Verification items for the finished model (mm, model axes). Face numbers are marked on the shaded views. A direction names the side the tool comes from. Round coordinates to 2 decimals unless told otherwise and drop trailing zeros. Write each loop counter-clockwise with the first axis right and the second up, starting at its lowest first coordinate (ties: lowest second). Pieces come first, ordered by that corner, then holes. Notation, with made-up numbers: M -17.75,3 L -6.75,3 A28 cw -6.75,41 Z; hole C 77.5,12 d9. An arc over 180 degrees is marked long. One line per item, written item: value. Start each with the question number.
from build123d import *

# Parameters (mm, degrees)
BASE_FLANGE1_DEPTH             = 7.62
EDGE_FLANGE1_STRIP_W           = 12.7
EDGE_FLANGE1_STRIP_H           = 1.5875
EDGE_FLANGE1_STRIP_CUT_DEPTH   = 13.689174868
EDGE_FLANGE1_STRIP_2_W         = 12.7
EDGE_FLANGE1_STRIP_2_H         = 1.5875
EDGE_FLANGE1_STRIP_CUT_2_DEPTH = 13.689174868
EDGE_FLANGE1_DEPTH             = 13.689174868
EDGE_FLANGE1_BEND_DEPTH        = 13.689174868
SKETCH12_W                     = 0.396875
SKETCH12_H                     = 4.784490506
SKETCH12_H_2                   = 4.782978668
CUT_EXTRUDE3_DEPTH             = 25.4
SKETCH13_W                     = 0.396875
SKETCH13_H                     = 4.7625
CUT_EXTRUDE4_DEPTH             = 25.4
FILLET2_R                      = 0.79375
BOSS_EXTRUDE1_DEPTH            = 1.5875
FILLET3_R                      = 3.175
FILLET4_R                      = 4.7625
FILLET5_R                      = 0.79375


# Read off the part's stored shape, not the designer's step: Base-Flange1
# Sheet-metal steps are written as plain solids
with BuildPart() as part:
    # Base-Flange1 outline → Base-Flange1 (new body)
    with BuildSketch(Plane(origin=(0, 0, 0), x_dir=(1, 0, 0), z_dir=(0, 1, 0))):
        with BuildLine():
            ThreePointArc((24.665208878, -10.952288676), (26.30984284, -6.00976921), (26.974319291, -0.843359375))
            Line((26.974319291, -0.843359375), (25.387594627, -0.79375))
            ThreePointArc((25.387594627, -0.79375), (24.762205026, -5.656253374), (23.214314238, -10.308036401))
            ThreePointArc((23.214314238, -10.308036401), (22.645724221, -11.325105064), (21.900863739, -12.221155361))
            Line((21.900863739, -12.221155361), (12.221155361, -21.900863739))
            ThreePointArc((12.221155361, -21.900863739), (11.325105064, -22.645724221), (10.308036401, -23.214314238))
            ThreePointArc((10.308036401, -23.214314238), (0, -25.4), (-10.308036401, -23.214314238))
            ThreePointArc((-10.308036401, -23.214314238), (-11.325105064, -22.645724221), (-12.221155361, -21.900863739))
            Line((-12.221155361, -21.900863739), (-21.900863739, -12.221155361))
            ThreePointArc((-21.900863739, -12.221155361), (-22.645724221, -11.325105064), (-23.214314238, -10.308036401))
            ThreePointArc((-23.214314238, -10.308036401), (-24.762205026, -5.656253374), (-25.387594627, -0.79375))
            Line((-25.387594627, -0.79375), (-26.974319291, -0.843359375))
            ThreePointArc((-26.974319291, -0.843359375), (-26.30984284, -6.00976921), (-24.665208878, -10.952288676))
            ThreePointArc((-24.665208878, -10.952288676), (-23.954471356, -12.223624504), (-23.023395754, -13.343687376))
            Line((-23.023395754, -13.343687376), (-13.343687376, -23.023395754))
            ThreePointArc((-13.343687376, -23.023395754), (-12.223624504, -23.954471356), (-10.952288676, -24.665208878))
            ThreePointArc((-10.952288676, -24.665208878), (0, -26.9875), (10.952288676, -24.665208878))
            ThreePointArc((10.952288676, -24.665208878), (12.223624504, -23.954471356), (13.343687376, -23.023395754))
            Line((13.343687376, -23.023395754), (23.023395754, -13.343687376))
            ThreePointArc((23.023395754, -13.343687376), (23.954471356, -12.223624504), (24.665208878, -10.952288676))
        make_face()
    extrude(amount=BASE_FLANGE1_DEPTH)

    # Edge-Flange1 strip (across the edge) → Edge-Flange1 strip cut (cut)
    with BuildSketch(Plane(origin=(-23.023395754, 0, 13.343687376), x_dir=(0, 1, 0), z_dir=(0.7071067811865437, 0, 0.7071067811865515))):
        with Locations((-1.5875, -0.79375)):
            Rectangle(EDGE_FLANGE1_STRIP_W, EDGE_FLANGE1_STRIP_H)
    extrude(amount=EDGE_FLANGE1_STRIP_CUT_DEPTH, mode=Mode.SUBTRACT)

    # Edge-Flange1 strip 2 (across the edge) → Edge-Flange1 strip cut 2 (cut)
    with BuildSketch(Plane(origin=(13.343687376, 0, 23.023395754), x_dir=(0, 1, 0), z_dir=(0.7071067811865512, 0, -0.7071067811865438))):
        with Locations((-1.5875, -0.79375)):
            Rectangle(EDGE_FLANGE1_STRIP_2_W, EDGE_FLANGE1_STRIP_2_H)
    extrude(amount=EDGE_FLANGE1_STRIP_CUT_2_DEPTH, mode=Mode.SUBTRACT)

    # Edge-Flange1 section (across the edge) → Edge-Flange1 (add)
    with BuildSketch(Plane(origin=(-23.023395754, 0, 13.343687376), x_dir=(0, 1, 0), z_dir=(0.7071067811865437, 0, 0.7071067811865515))):
        with BuildLine():
            Line((0, 3.175), (0, 7.9375))
            Line((0, 7.9375), (1.5875, 7.9375))
            Line((1.5875, 7.9375), (1.5875, 3.175))
            ThreePointArc((1.5875, 3.175), (2.51743597, 0.92993597), (4.7625, 0))
            Line((4.7625, 0), (4.7625, -1.5875))
            ThreePointArc((4.7625, -1.5875), (1.394903955, -0.192596045), (0, 3.175))
        make_face()
    extrude(amount=EDGE_FLANGE1_DEPTH)

    # Edge-Flange1 section 2 (across the edge) → Edge-Flange1 bend (add)
    with BuildSketch(Plane(origin=(13.343687376, 0, 23.023395754), x_dir=(0, 1, 0), z_dir=(0.7071067811865512, 0, -0.7071067811865438))):
        with BuildLine():
            Line((0, 3.175), (0, 7.9375))
            Line((0, 7.9375), (1.5875, 7.9375))
            Line((1.5875, 7.9375), (1.5875, 3.175))
            ThreePointArc((1.5875, 3.175), (2.51743597, 0.92993597), (4.7625, 0))
            Line((4.7625, 0), (4.7625, -1.5875))
            ThreePointArc((4.7625, -1.5875), (1.394903955, -0.192596045), (0, 3.175))
        make_face()
    extrude(amount=EDGE_FLANGE1_BEND_DEPTH)

    # Sketch12 → Cut-Extrude3 (cut)
    with BuildSketch(Plane(origin=(-23.796201641, 0, 23.796201641), x_dir=(0.7071067811865438, 3.532708032038459e-15, 0.7071067811865512), z_dir=(-0.7071067811865512, -3.532708032038497e-15, 0.7071067811865438))):
        with Locations((7.043024934, 2.370254747)):
            Rectangle(SKETCH12_W, SKETCH12_H)
        with Locations((-7.043024934, 2.371010666)):
            Rectangle(SKETCH12_W, SKETCH12_H_2)
    extrude(amount=-CUT_EXTRUDE3_DEPTH, mode=Mode.SUBTRACT)

    # Sketch13 → Cut-Extrude4 (cut)
    with BuildSketch(Plane(origin=(23.796201641, 0, 23.796201641), x_dir=(0.7071067811865513, 3.414951097637176e-15, -0.7071067811865437), z_dir=(0.7071067811865437, -3.414951097637212e-15, 0.7071067811865513))):
        with Locations((7.043024934, 2.38125)):
            Rectangle(SKETCH13_W, SKETCH13_H)
        with Locations((-7.043024934, 2.38125)):
            Rectangle(SKETCH13_W, SKETCH13_H)
    extrude(amount=-CUT_EXTRUDE4_DEPTH, mode=Mode.SUBTRACT)

    # Fillet2
    fillet2_edges = [part.edges().sort_by_distance(p)[0] for p in [
        (-12.493889076, 0, 22.734863462),
        (-22.734863462, 0, 12.493889076),
        (-26.180956959, 0, 0.818554688),
        (22.734863462, 0, 12.493889076),
        (26.180956959, 0, 0.818554688),
        (12.493889076, 0, 22.734863462),
        (-26.180956959, 7.62, 0.818554688),
        (26.180956959, 7.62, 0.818554688),
    ]]
    fillet(fillet2_edges, radius=FILLET2_R)

    # Sketch4 → Boss-Extrude1 (add)
    # profile 1 of 2: a face of its own
    with BuildSketch(Plane(origin=(0, 1.5875, 0), x_dir=(1, 0, 0), z_dir=(0, 1, 0))):
        Polygon((-18.956347452, -28.63605583), (-25.46851022, -35.148218598), (-16.119559737, -44.49716908), (-27.344879889, -55.722489231), (-55.722489231, -27.344879889), (-44.49716908, -16.119559737), (-35.148218598, -25.46851022), (-28.63605583, -18.956347452), align=None)
        Polygon((-48.268876651, -28.063300378), (-28.063300378, -48.268876651), (-25.818236348, -46.02381262), (-46.02381262, -25.818236348), align=None, mode=Mode.SUBTRACT)
    # profile 2 of 2: a face of its own
    with BuildSketch(Plane(origin=(0, 1.5875, 0), x_dir=(1, 0, 0), z_dir=(0, 1, 0))):
        Polygon((18.956347452, -28.63605583), (25.46851022, -35.148218598), (16.119559737, -44.49716908), (27.344879889, -55.722489231), (55.722489231, -27.344879889), (44.49716908, -16.119559737), (35.148218598, -25.46851022), (28.63605583, -18.956347452), align=None)
        Polygon((29.185832393, -49.391408666), (26.940768363, -47.146344636), (47.146344636, -26.940768363), (49.391408666, -29.185832393), align=None, mode=Mode.SUBTRACT)
    extrude(amount=-BOSS_EXTRUDE1_DEPTH)

    # Fillet3
    fillet3_edges = [part.edges().sort_by_distance(p)[0] for p in [
        (-16.119559737, 0.79375, 44.49716908),
        (-27.344879889, 0.79375, 55.722489231),
        (-55.722489231, 0.79375, 27.344879889),
        (-44.49716908, 0.79375, 16.119559737),
        (44.49716908, 0.79375, 16.119559737),
        (55.722489231, 0.79375, 27.344879889),
        (27.344879889, 0.79375, 55.722489231),
        (16.119559737, 0.79375, 44.49716908),
    ]]
    fillet(fillet3_edges, radius=FILLET3_R)

    # Fillet4
    fillet4_edges = [part.edges().sort_by_distance(p)[0] for p in [
        (-25.46851022, 0.79375, 35.148218598),
        (-35.148218598, 0.79375, 25.46851022),
        (35.148218598, 0.79375, 25.46851022),
        (25.46851022, 0.79375, 35.148218598),
    ]]
    fillet(fillet4_edges, radius=FILLET4_R)

    # Fillet5
    fillet5_edges = [part.edges().sort_by_distance(p)[0] for p in [
        (-46.02381262, 0.79375, 25.818236348),
        (-25.818236348, 0.79375, 46.02381262),
        (-28.063300378, 0.79375, 48.268876651),
        (-48.268876651, 0.79375, 28.063300378),
        (29.185832393, 0.79375, 49.391408666),
        (26.940768363, 0.79375, 47.146344636),
        (47.146344636, 0.79375, 26.940768363),
        (49.391408666, 0.79375, 29.185832393),
    ]]
    fillet(fillet5_edges, radius=FILLET5_R)


solid = part.part
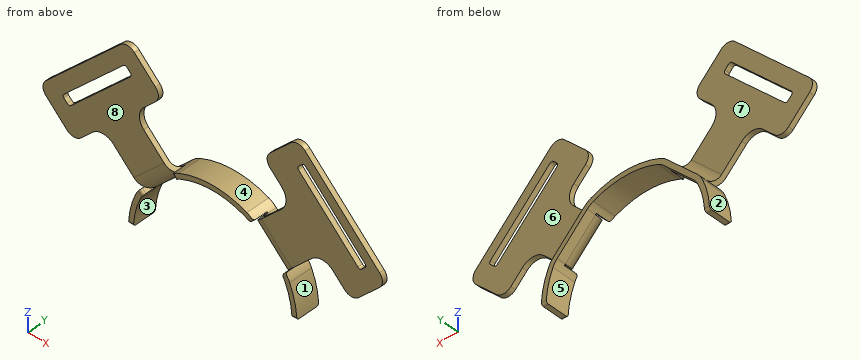
1) Mould release check, pull along X, two halves, no side actions. Record for the marked faces 1, 2 and 3: pulls with the +X half, pulls with the -X half, needs draft (parallel to the pull), parting line crosses it, or undercut.
2) Cross-section at D-D (z = 36.5). Record the boundary of the cut face in (x, y).
3) Cross-section at B-B (x = -33). Record the boundary of the cut face in (y, z), then the cut area to 3 significant figures.
4) Cross-section at A-A (z = 4.5). Record the boundary of the cut face in (x, y).
5) Gauge pin test, flat ends, axial feed: pin 1 Ø19.5 at (x, z) = (-41, 40.5) entering from +Y; pin 2 Ø1.1 at (x, z) = (23, 12.5) entering from -Y; pin 3 Ø6 at (x, z) = (1, 31) entering from +Y. Record the tip position at first contact, or that the pin passes through.
6) Access from +Z, -Z, +X, -X, +Y, -Y to the whole of each face (thin tool, end or side, straight path). Record for the marked faces 4, 5, 6, 7 and 8.
7) Thickness scan on line 1 (Y direction, x = 26, z = 32); line 2 (X direction, y = 5.75, z = 13.5); line 3 (X direction, y = 6.25, z = 19). Record the ranges inside material, lowest first.
8) Cross-section at C-C (y = 3.25). State how many separate pieces and enclosed holes the cut face has, then the cut area to 3 significant figures.
Results below:
1. face 1: pulls with the +X half
1. face 2: pulls with the -X half
1. face 3: undercut
2. outline: M -46.57,0 L -39.83,0 L -39.83,1.59 L -46.57,1.59 Z; M -35.34,0 L -23.3,0 L -23.3,1.59 L -35.34,1.59 Z; M 23.3,0 L 37.59,0 L 37.59,1.59 L 23.3,1.59 Z; M 42.08,0 L 46.57,0 L 46.57,1.59 L 42.08,1.59 Z
3. outline: M 0,22.98 L 1.59,22.98 L 1.59,38.84 L 0,38.84 Z; M 0,43.33 L 1.59,43.33 L 1.59,50.07 L 0,50.07 Z
3. area: 35.9 mm²
4. outline: M -26.61,0 L -25,0 L -25,7.62 L -26.61,7.62 Z; M 25,0 L 26.61,0 L 26.61,7.62 L 25,7.62 Z
5. pin 1: stops at y = 1.59
5. pin 2: stops at y = 0
5. pin 3: passes through
6. face 4: +Z, +Y, -Y
6. face 5: -Z, +Y, -Y
6. face 6: +Z, +X, +Y
6. face 7: +Z, -X, +Y
6. face 8: +Z, -Z, +X, -X, -Y
7. line 1: y = 0 to 1.59
7. line 2: x = -22.87 to -20.62, 20.62 to 22.87
7. line 3: x = -17.37 to -15.12, 15.12 to 17.37
8. separate pieces: 5
8. enclosed holes: 0
8. area: 128 mm²
